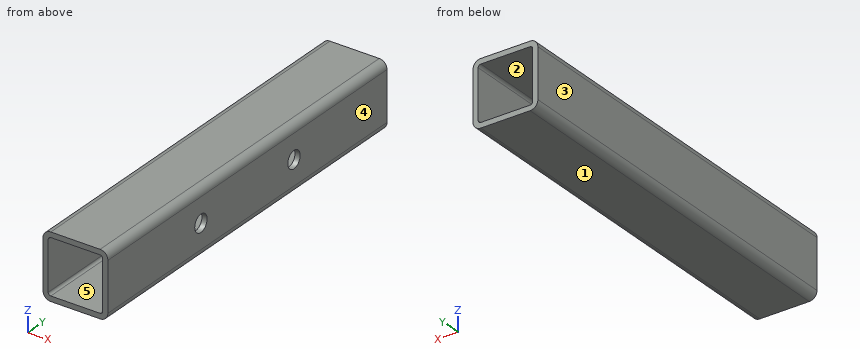
Autodesk Inventor part; units mm, degrees
ref_plane "XZ Plane" through (0, 0, 0) normal (0, 1, 0) x (-1, 0, 0)
sketch "Sketch1" plane through (0, 0, 0) normal (0, 1, 0) x (-1, 0, 0)
  line L0 (-9.5, 11.5) -> (9.5, 11.5) construction
  line L1 (11.5, 9.5) -> (11.5, -9.5) construction
  line L2 (9.5, -11.5) -> (-9.5, -11.5) construction
  line L3 (-11.5, -9.5) -> (-11.5, 9.5) construction
  line L4 (-11.5, 11.5) -> (11.5, -11.5) construction
  line L5 (11.5, 11.5) -> (-11.5, -11.5) construction
  arc A0 (11.5, 9.5) -> (9.5, 11.5) centre (9.5, 9.5) ccw construction
  arc A1 (9.5, -11.5) -> (11.5, -9.5) centre (9.5, -9.5) ccw construction
  arc A2 (-11.5, -9.5) -> (-9.5, -11.5) centre (-9.5, -9.5) ccw construction
  arc A3 (-9.5, 11.5) -> (-11.5, 9.5) centre (-9.5, 9.5) ccw construction
  line L6 (-9.5, -12.5) -> (9.5, -12.5)
  arc A4 (9.5, -12.5) -> (12.5, -9.5) centre (9.5, -9.5) ccw
  line L7 (12.5, -9.5) -> (12.5, 9.5)
  arc A5 (12.5, 9.5) -> (9.5, 12.5) centre (9.5, 9.5) ccw
  line L8 (9.5, 12.5) -> (-9.5, 12.5)
  arc A6 (-9.5, 12.5) -> (-12.5, 9.5) centre (-9.5, 9.5) ccw
  line L9 (-12.5, 9.5) -> (-12.5, -9.5)
  arc A7 (-12.5, -9.5) -> (-9.5, -12.5) centre (-9.5, -9.5) ccw
  line L10 (10.5, -9.5) -> (10.5, 9.5)
  arc A8 (10.5, 9.5) -> (9.5, 10.5) centre (9.5, 9.5) ccw
  line L11 (9.5, 10.5) -> (-9.5, 10.5)
  arc A9 (-9.5, 10.5) -> (-10.5, 9.5) centre (-9.5, 9.5) ccw
  line L12 (-10.5, 9.5) -> (-10.5, -9.5)
  arc A10 (-10.5, -9.5) -> (-9.5, -10.5) centre (-9.5, -9.5) ccw
  line L13 (-9.5, -10.5) -> (9.5, -10.5)
  arc A11 (9.5, -10.5) -> (10.5, -9.5) centre (9.5, -9.5) ccw
  point P0 (0, 0)
  point P1 (0, 0)
  point P2 (0, 0)
  dimension "d10" = 2
  dimension "depth" = 25
  dimension "width" = 25
  dimension "thickness" = 2
extrude "Extrusion1" add sketch "Sketch1" along normal blind 150
sketch "Sketch2" plane through (12.5, 0, 9.5) normal (1, 0, 0) x (0, 0, -1)
  line L0 (9.5, -30) -> (9.5, 180) construction
  line L1 (0, 150) -> (19, 150)
  point P0 (9.5, 0)
  point P1 (9.5, 100)
  point P2 (9.5, 50)
  dimension "d16" = 50
  dimension "d17" = 50
hole "Hole1" at (12.5, 100, 0) at (12.5, 50, 0) direction (-1, 0, 0) diameter 6.647 depth 20.2 tip angle 118
equation "\"d10\" = thickness"
properties part number "Stopa v2 profil 1" material "Steel"
Could you check a few things on this model? Use its own coordinates, in mm. Face numbers are marked on the shaded views. A direction names the side the tool comes from. Round coordinates to 2 decimals unless told otherwise and drop trailing zeros. Order: outer loops, then holes, each group sorted by start corner. A loop starts at its lowest first (then second) coordinate and runs counter-clockwise, first axis right, second up. Notation, with made-up numbers: M -38,36 L 21,36 A11 cw 21,52 Z; hole C -3,-24.5 d3. An arc over 180 degrees is marked long. One line per item, written item: value.
(1) Imagine slicing it at D-D (z = -6.25). Write out the boundary of the cut face in (x, y), and give its area (3 significant figures).
Ans:
outline: M -12.5,0 L -10.5,0 L -10.5,150 L -12.5,150 Z; M 10.5,0 L 12.5,0 L 12.5,150 L 10.5,150 Z
area: 600 mm^2
(2) If we mould it in two halves opening along X, with no side actions, what happens to the marked faces 1, 2 and 3? For each: released by +X, released by -X, zero draft, split by the parting line, or undercut.
Ans:
face 1: zero draft
face 2: undercut
face 3: released by -X
(3) Imagine slicing it at B-B (z = 0). Write out the boundary of the cut face in (x, y), and give its area (3 significant figures).
Ans:
outline: M -12.5,0 L -10.5,0 L -10.5,150 L -12.5,150 Z; M 10.5,0 L 12.5,0 L 12.5,46.68 L 10.5,46.68 Z; M 10.5,53.32 L 12.5,53.32 L 12.5,96.68 L 10.5,96.68 Z; M 10.5,103.32 L 12.5,103.32 L 12.5,150 L 10.5,150 Z
area: 573 mm^2
(4) Which directions (+Z, -Z, +X, -X, +Y, -Y) give clear straight access to the entire face, cutting with the end or side of a thin tool? Please do the marked faces 4 and 5.
Ans:
face 4: +Z, -Z, +X, +Y, -Y
face 5: +Y, -Y
(5) I'm going to push a flat-ended pin straight in: P1, Ø10, axis at x = 8.5, z = -3.5, coming from the +Y side. Where does the tip first touch, or does it pass through?
Ans:
P1: stops at y = 150
(6) I need wall thicknesses on line 1 along Y through (x, z) = (12.1, 0); line 2 along Z through (x, y) = (0.75, 13.5). Which ranges of each line are inside material? Lowest first, please. Write a range as from..to.
Ans:
line 1: y = 0..46.68, 53.32..96.68, 103.32..150
line 2: z = -12.5..-10.5, 10.5..12.5
(7) Imagine slicing it at C-C (y = 92). Write out the boundary of the cut face in (x, z), and give its area (3 significant figures).
Ans:
outline: M -12.5,-9.5 A3 ccw -9.5,-12.5 L 9.5,-12.5 A3 ccw 12.5,-9.5 L 12.5,9.5 A3 ccw 9.5,12.5 L -9.5,12.5 A3 ccw -12.5,9.5 Z; hole M -10.5,-9.5 A1 ccw -9.5,-10.5 L 9.5,-10.5 A1 ccw 10.5,-9.5 L 10.5,9.5 A1 ccw 9.5,10.5 L -9.5,10.5 A1 ccw -10.5,9.5 Z
area: 177 mm^2
(8) Imagine slicing it at A-A (x = -3.75). Write out the boundary of the cut face in (y, z), and give its area (3 significant figures).
Ans:
outline: M 0,-12.5 L 150,-12.5 L 150,-10.5 L 0,-10.5 Z; M 0,10.5 L 150,10.5 L 150,12.5 L 0,12.5 Z
area: 600 mm^2
